Job drawing, mm, ordinate dimensions from the low corner. One solid piece. A direction names the side the tool comes from. Round coordinates to 2 decimals unless told otherwise and drop trailing zeros. Loops run counter-clockwise (first coordinate to the right, second up) from the corner with the lowest first, then second, coordinate; pieces in that order, holes last.
1) Band-saw the part on C-C, the plane y = 118. Write the cut outline in (x, z).
2) 3-axis set-ups, long thin cutter, end or side, ignore diameter. For the marked faces 1 and 2: which of +Z, -Z, +X, -X, +Y, -Y reach the whole face in a straight line?
3) Band-saw the part on D-D, the plane z = 39.5. Write the cut outline in (x, y).
4) Drop flat-ended pins along their axis: P1, Ø3.5, axis at x = 20.5, y = 1, coming from the +Z side; P2, Ø0.9, axis at y = 2, z = 56, coming from the -X side; P3, Ø0.9, axis at y = 1.5, z = 49.5, coming from the +X side. Give the stop position or say it passes through.
5) Band-saw the part on B-B, the plane x = 16. Write the cut outline in (y, z).
6) Band-saw the part on A-A, the plane z = 66. Write the cut outline in (x, y).
7) Probe line 1 (Z direction, x = 64.5, y = 116.5); line 2 (Y direction, x = 65, z = 77); line 3 (Y direction, x = 20, z = 8). List the from-to ranges inside material, lowest first.
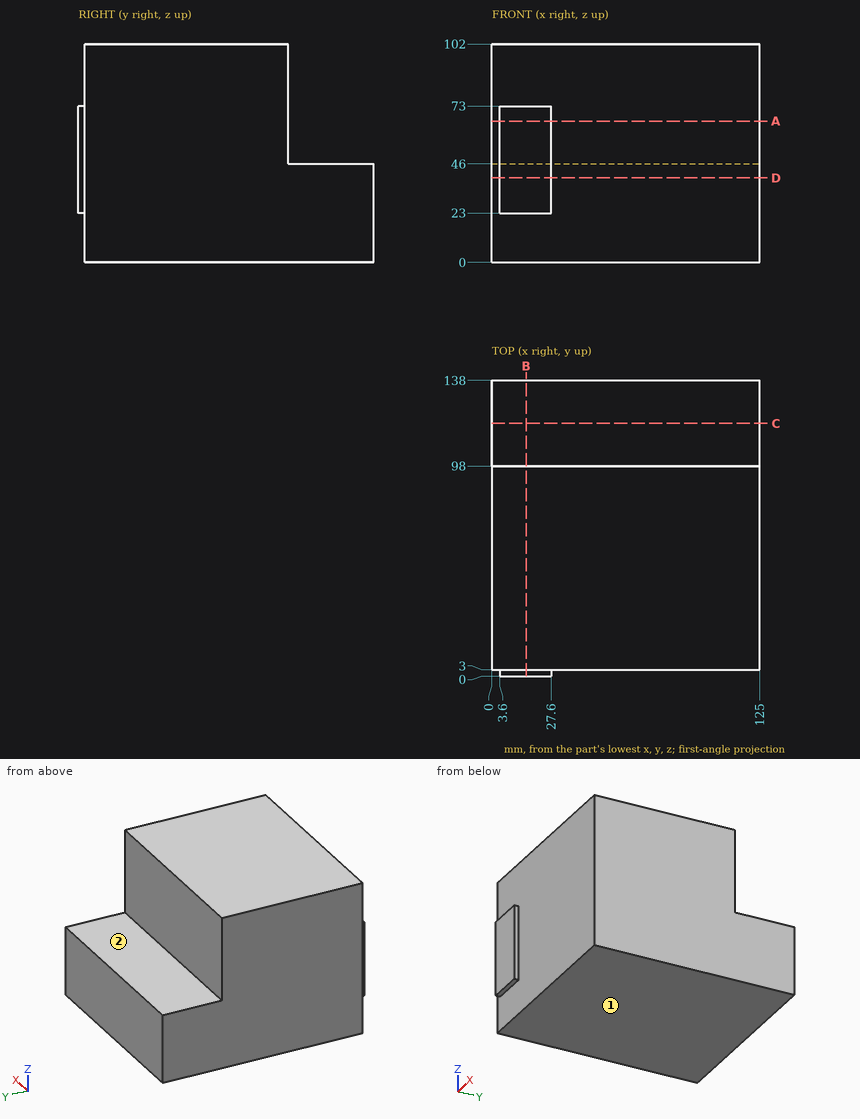
Reported:
1. outline: (0, 0) - (125, 0) - (125, 46) - (0, 46) - close
2. face 1: -Z, +X, -X, +Y, -Y
2. face 2: +Z, +X, -X, +Y
3. outline: (0, 3) - (3.6, 3) - (3.6, 0) - (27.6, 0) - (27.6, 3) - (125, 3) - (125, 138) - (0, 138) - close
4. P1: stops at z = 73
4. P2: stops at x = 3.6
4. P3: stops at x = 27.6
5. outline: (0, 23) - (3, 23) - (3, 0) - (138, 0) - (138, 46) - (98, 46) - (98, 102) - (3, 102) - (3, 73) - (0, 73) - close
6. outline: (0, 3) - (3.6, 3) - (3.6, 0) - (27.6, 0) - (27.6, 3) - (125, 3) - (125, 98) - (0, 98) - close
7. line 1: z = 0 to 46
7. line 2: y = 3 to 98
7. line 3: y = 3 to 138
